from build123d import *

# Parameters (mm, degrees)
SKETCH_1_W          = 38
SKETCH_1_H          = 5
SKETCH_1_R          = 0.95
EXTRUDE_1_DEPTH     = 2
EXTRUDE_2_DEPTH     = 38
SKETCH_3_R          = 0.95
CUT_EXTRUDE_1_DEPTH = 12


with BuildPart() as part:
    # 草图1 → 凸台-拉伸1 (new body)
    with BuildSketch(Plane.XY):
        with Locations((19, -2.5)):
            Rectangle(SKETCH_1_W, SKETCH_1_H)
        with Locations((31.35, -2.5)):
            Circle(SKETCH_1_R, mode=Mode.SUBTRACT)
    extrude(amount=EXTRUDE_1_DEPTH)

    # 草图2 → 凸台-拉伸2 (add)
    with BuildSketch(Plane(origin=(38, 0, 0), x_dir=(0, 0, -1), z_dir=(1, 0, 0))):
        Polygon((0, 0), (-2, 5), (-4, 5), (-2, 0), align=None)
    extrude(amount=-EXTRUDE_2_DEPTH)

    # 草图3 → 切除-拉伸1 (cut)
    with BuildSketch(Plane.XY.offset(2)):
        with Locations((21.35, -2.5)):
            Circle(SKETCH_3_R)
    extrude(amount=-CUT_EXTRUDE_1_DEPTH, mode=Mode.SUBTRACT)


solid = part.part
CAD build for the part. Positions are in the model's coordinates, mm. Give positions to 0.01 mm unless a question says otherwise; leave off trailing zeros. Write each loop counter-clockwise with the first axis right and the second up, starting at its lowest first coordinate (ties: lowest second). Pieces come first, ordered by that corner, then holes. Notation, with made-up numbers: (-36.75, 44.5) - (19.25, 44.5) arc R6 cw to (19.25, 55.5) - close; hole circle Ø9 at (17.25, -3). An arc over 180 degrees is marked (long way). Put each result on its own line as item: value.
(1) Wall check: L1, parallel to Z at x = 23, y = -2.75; L2, parallel to Y at x = 31.35, z = 0.45 (3 decimals); L3, parallel to Y at x = 29, z = 2.5. Give the ranges that are in metal, low to high.
Working result:
L1: 0 to 2
L2: -5 to -3.45, -1.55 to 1.125
L3: 1.25 to 5
(2) Drop flat-ended pins along their axis: pin 1 Ø2 at (x, z) = (21, 3.5) entering from -Y; pin 2 Ø5.5 at (x, y) = (21.5, -3) entering from +Z. Give the stop position or say it passes through.
Working result:
pin 1: y = 1.25
pin 2: z = 2
(3) Saw through at C-C (z = 1.5). List the corners of the cut face in (x, y).
Working result:
outline: (0, -5) - (38, -5) - (38, 3.75) - (0, 3.75) - close; hole circle Ø1.9 at (21.35, -2.5); hole circle Ø1.9 at (31.35, -2.5)
(4) Pull direction Y, two halves, no side cores. Call faces 1 (the flat face through (19, -2, 2)), 2 (the flat face through (19.3, 2.5, 3)), 3 (the cylindrical face through (30.4, -2.5, 1)): released by +Y, released by -Y, zero draft, split by the parting line, or undercut.
Working result:
face 1: zero draft
face 2: released by -Y
face 3: undercut
(5) Saw through at D-D (x = 6.5). List the corners of the cut face in (y, z).
Working result:
outline: (-5, 0) - (0, 0) - (5, 2) - (5, 4) - (0, 2) - (-5, 2) - close
(6) Saw through at A-A (y = -2.5). List the corners of the cut face in (x, z), then the cut area to 3 significant figures.
Working result:
outline: (0, 0) - (20.4, 0) - (20.4, 2) - (0, 2) - close; (22.3, 0) - (30.4, 0) - (30.4, 2) - (22.3, 2) - close; (32.3, 0) - (38, 0) - (38, 2) - (32.3, 2) - close
area: 68.4 mm^2
(7) Saw through at B-B (x = 21.35). List the corners of the cut face in (y, z).
Working result:
outline: (-5, 0) - (-3.45, 0) - (-3.45, 2) - (-5, 2) - close; (-1.55, 0) - (0, 0) - (5, 2) - (5, 4) - (0, 2) - (-1.55, 2) - close
